Read the model definition and answer for the solid it produces. Units are mm, in the model's axes. A direction names the side the tool comes from. Round coordinates to 2 decimals unless told otherwise and drop trailing zeros. Write each loop counter-clockwise with the first axis right and the second up, starting at its lowest first coordinate (ties: lowest second). Pieces come first, ordered by that corner, then holes.
from build123d import *

# Parameters (mm, degrees)
CROQUIS1_R              = 27.5
SALIENTE_EXTRUIR1_DEPTH = 40
CROQUIS2_R              = 11.800520357
CORTAR_EXTRUIR1_DEPTH   = 15
CORTAR_EXTRUIR4_START   = 15
CROQUIS3_R              = 11.800520357
CORTAR_EXTRUIR4_DEPTH   = 15


with BuildPart() as part:
    # Croquis1 → Saliente-Extruir1 (new body)
    with BuildSketch(Plane.XY):
        Circle(CROQUIS1_R)
    extrude(amount=SALIENTE_EXTRUIR1_DEPTH)

    # Croquis2 → Cortar-Extruir1 (cut)
    with BuildSketch(Plane.ZY.offset(27.5)):
        with Locations((20, 0)):
            Circle(CROQUIS2_R)
    extrude(amount=-CORTAR_EXTRUIR1_DEPTH, mode=Mode.SUBTRACT)

    # Croquis3 → Cortar-Extruir4 (cut)
    with BuildSketch(Plane.ZY.offset(-27.5).offset(CORTAR_EXTRUIR4_START)):
        with Locations((20, 0)):
            Circle(CROQUIS3_R)
    extrude(amount=-CORTAR_EXTRUIR4_DEPTH, mode=Mode.SUBTRACT)


solid = part.part
Q1. Section D-D (y = -9) is taken. Determine the outline of the cut face in (x, z), then the cut area to 3 significant figures.
Verdict:
outline: (-25.99, 0) - (25.99, 0) - (25.99, 12.37) - (12.5, 12.37) - (12.5, 27.63) - (25.99, 27.63) - (25.99, 40) - (-25.99, 40) - (-25.99, 27.63) - (-12.5, 27.63) - (-12.5, 12.37) - (-25.99, 12.37) - close
area: 1,670 mm2
Q2. Section C-C (z = 20) is taken. Determine the outline of the cut face in (x, y).
Verdict:
outline: (-24.84, -11.8) arc R27.5 ccw to (24.84, -11.8) - (12.5, -11.8) - (12.5, 11.8) - (24.84, 11.8) arc R27.5 ccw to (-24.84, 11.8) - (-12.5, 11.8) - (-12.5, -11.8) - close
Q3. Section A-A (y = 0) is taken. Determine the outline of the cut face in (x, z).
Verdict:
outline: (-27.5, 0) - (27.5, 0) - (27.5, 8.2) - (12.5, 8.2) - (12.5, 31.8) - (27.5, 31.8) - (27.5, 40) - (-27.5, 40) - (-27.5, 31.8) - (-12.5, 31.8) - (-12.5, 8.2) - (-27.5, 8.2) - close
Q4. Section B-B (x = -16.5) is taken. Determine the outline of the cut face in (y, z), then the cut area to 3 significant figures.
Verdict:
outline: (-22, 0) - (22, 0) - (22, 40) - (-22, 40) - close; hole circle Ø23.6 at (0, 20)
area: 1,320 mm2
Q5. Flat-ended cylindrical pins translate along their axes: pin 1 Ø8 at (y, z) = (-11.5, 34.5) entering from +X; pin 2 Ø5 at (y, z) = (-3, 16) entering from +X; pin 3 Ø1.5 at (x, y) = (-16, 3.5) entering from -Z; pin 4 Ø1.5 at (y, z) = (-18.5, 7.5) entering from -X. Find the tip coordinate at first contact, or state that the pin passes through.
Verdict:
pin 1: stops at x = 26.46
pin 2: stops at x = 12.5
pin 3: stops at z = 0
pin 4: stops at x = -21
Q6. Which of the six approach directions +Z, -Z, +X, -X, +Y, -Y give full straight-line access (tool end or side, diameter ignored) to faces 1 (the flat face through (0, 0, 40)), 2 (the flat face through (-12.5, 0, 20)), 3 (the flat face through (12.5, 0, 20))?
Verdict:
face 1: +Z, +X, -X, +Y, -Y
face 2: -X
face 3: +X
Q7. Straight lines are drawn through the part: probe 1 along Z at (x, y) = (24.5, 8.5); probe 2 along Y at (x, z) = (-17, 30.5); probe 3 along Y at (x, z) = (-14.5, 12). For each, find the intervals that lie inside material, in ascending order.
Verdict:
probe 1: z = 0 to 11.81, 28.19 to 40
probe 2: y = -21.62 to -5.39, 5.39 to 21.62
probe 3: y = -23.37 to -8.67, 8.67 to 23.37
